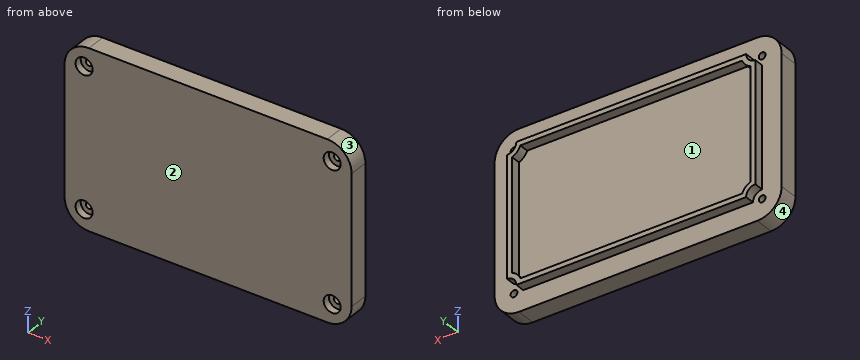
from build123d import *

# Parameters (mm, degrees)
SKETCH1_R           = 1.4
BOSS_EXTRUDE1_DEPTH = 8
BOSS_EXTRUDE2_DEPTH = 8
BOSS_EXTRUDE3_DEPTH = 4
SKETCH4_R           = 3.5
CUT_EXTRUDE1_DEPTH  = 3


with BuildPart() as part:
    # Sketch1 → Boss-Extrude1 (new body)
    with BuildSketch(Plane(origin=(0, 0, 0), x_dir=(1, 0, 0), z_dir=(0, 1, 0))):
        with BuildLine():
            ThreePointArc((-49, 36.5), (-56.071067812, 33.571067812), (-59, 26.5))
            Line((-59, 26.5), (-59, -26.5))
            ThreePointArc((-59, -26.5), (-56.071067812, -33.571067812), (-49, -36.5))
            Line((-49, -36.5), (49, -36.5))
            ThreePointArc((49, -36.5), (56.071067812, -33.571067812), (59, -26.5))
            Line((59, -26.5), (59, 26.5))
            ThreePointArc((59, 26.5), (56.071067812, 33.571067812), (49, 36.5))
            Line((49, 36.5), (-49, 36.5))
        make_face()
        with Locations(Location((-51, -28.5, 0), (0, 0, 270))):
            Circle(SKETCH1_R, mode=Mode.SUBTRACT)
        with Locations(Location((51, -28.5, 0), (0, 0, 270))):
            Circle(SKETCH1_R, mode=Mode.SUBTRACT)
        with Locations(Location((-51, 28.5, 0), (0, 0, 270))):
            Circle(SKETCH1_R, mode=Mode.SUBTRACT)
        with BuildLine():
            Line((43.828427125, -28.5), (-43.828427125, -28.5))
            Line((-43.828427125, -28.5), (-47.234932778, -28.5))
            ThreePointArc((-47.234932778, -28.5), (-48.337695436, -25.837695436), (-51, -24.734932778))
            Line((-51, -24.734932778), (-51, -21.328427125))
            Line((-51, -21.328427125), (-51, 21.328427125))
            Line((-51, 21.328427125), (-51, 24.734932778))
            ThreePointArc((-51, 24.734932778), (-48.337695436, 25.837695436), (-47.234932778, 28.5))
            Line((-47.234932778, 28.5), (-43.828427125, 28.5))
            Line((-43.828427125, 28.5), (43.828427125, 28.5))
            Line((43.828427125, 28.5), (47.234932778, 28.5))
            ThreePointArc((47.234932778, 28.5), (48.337695436, 25.837695436), (51, 24.734932778))
            Line((51, 24.734932778), (51, 21.328427125))
            Line((51, 21.328427125), (51, -21.328427125))
            Line((51, -21.328427125), (51, -24.734932778))
            ThreePointArc((51, -24.734932778), (48.337695436, -25.837695436), (47.234932778, -28.5))
            Line((47.234932778, -28.5), (43.828427125, -28.5))
        make_face(mode=Mode.SUBTRACT)
        with Locations(Location((51, 28.5, 0), (0, 0, 270))):
            Circle(SKETCH1_R, mode=Mode.SUBTRACT)
    extrude(amount=BOSS_EXTRUDE1_DEPTH)



with BuildPart() as body_2:
    # Sketch2 → Boss-Extrude2 (new body)
    with BuildSketch(Plane(origin=(0, 8, 0), x_dir=(1, 0, 0), z_dir=(0, 1, 0))):
        with BuildLine():
            Line((51, -24.734932778), (51, 24.734932778))
            ThreePointArc((51, 24.734932778), (48.337695436, 25.837695436), (47.234932778, 28.5))
            Line((47.234932778, 28.5), (-47.234932778, 28.5))
            ThreePointArc((-47.234932778, 28.5), (-48.337695436, 25.837695436), (-51, 24.734932778))
            Line((-51, 24.734932778), (-51, -24.734932778))
            ThreePointArc((-51, -24.734932778), (-48.337695436, -25.837695436), (-47.234932778, -28.5))
            Line((-47.234932778, -28.5), (47.234932778, -28.5))
            ThreePointArc((47.234932778, -28.5), (48.337695436, -25.837695436), (51, -24.734932778))
        make_face()
    extrude(amount=-BOSS_EXTRUDE2_DEPTH)


with BuildPart() as part_1:
    add(part.part)

    add(body_2.part)  # Boss-Extrude3 merges body 2
    # Sketch3 → Boss-Extrude3 (add)
    with BuildSketch(Plane(origin=(0, 8, 0), x_dir=(1, 0, 0), z_dir=(0, 1, 0))):
        with BuildLine():
            ThreePointArc((47.234932778, -28.5), (48.337695436, -25.837695436), (51, -24.734932778))
            Line((51, -24.734932778), (51, 24.734932778))
            ThreePointArc((51, 24.734932778), (48.337695436, 25.837695436), (47.234932778, 28.5))
            Line((47.234932778, 28.5), (-45.234932778, 28.5))
            Line((-45.234932778, 28.5), (-47.234932778, 28.5))
            ThreePointArc((-47.234932778, 28.5), (-48.337695436, 25.837695436), (-51, 24.734932778))
            Line((-51, 24.734932778), (-51, -24.734932778))
            ThreePointArc((-51, -24.734932778), (-48.337695436, -25.837695436), (-47.234932778, -28.5))
            Line((-47.234932778, -28.5), (47.234932778, -28.5))
        make_face()
        with BuildLine():
            ThreePointArc((-49, 23.092967535), (-46.923481873, 24.423481873), (-45.592967535, 26.5))
            Line((-45.592967535, 26.5), (45.592967535, 26.5))
            ThreePointArc((45.592967535, 26.5), (46.923481873, 24.423481873), (49, 23.092967535))
            Line((49, 23.092967535), (49, -23.092967535))
            ThreePointArc((49, -23.092967535), (46.923481873, -24.423481873), (45.592967535, -26.5))
            Line((45.592967535, -26.5), (-45.592967535, -26.5))
            ThreePointArc((-45.592967535, -26.5), (-46.923481873, -24.423481873), (-49, -23.092967535))
            Line((-49, -23.092967535), (-49, 23.092967535))
        make_face(mode=Mode.SUBTRACT)
    extrude(amount=BOSS_EXTRUDE3_DEPTH)

    # Sketch4 → Cut-Extrude1 (cut)
    with BuildSketch(Plane.XZ):
        with Locations(Location((-51, 28.5, 0), (0, 0, 270))):
            Circle(SKETCH4_R)
        with Locations(Location((51, 28.5, 0), (0, 0, 90))):
            Circle(SKETCH4_R)
        with Locations(Location((51, -28.5, 0), (0, 0, 270))):
            Circle(SKETCH4_R)
        with Locations(Location((-51, -28.5, 0), (0, 0, 90))):
            Circle(SKETCH4_R)
    extrude(amount=-CUT_EXTRUDE1_DEPTH, mode=Mode.SUBTRACT)


solid = part_1.part
CAD build for the part. Positions are in the model's coordinates, mm. Face numbers are marked on the shaded views. Give positions to 0.01 mm unless a question says otherwise; leave off trailing zeros. Write each loop counter-clockwise with the first axis right and the second up, starting at its lowest first coordinate (ties: lowest second). Pieces come first, ordered by that corner, then holes. Notation, with made-up numbers: M -38.75,87 L -33.75,87 A21 cw -33.75,122 Z; hole C 56,48 d11. An arc over 180 degrees is marked long. Put each result on its own line as item: value. Start each with the question number.
(1) Flat gauge pins, fed straight in: pin 1 Ø3 at (y, z) = (10.5, 10.5) entering from -X; pin 2 Ø2 at (x, y) = (20, 11) entering from +Z; pin 3 Ø2 at (x, z) = (-50.5, 27) entering from -Y. Where does each tip first touch, or does it go through?
(2) Band-saw the part on A-A, the plane y = 10.75. Write the cut outline in (x, z).
(3) Mould opens along Z. For the marked faces 1, 2, 3 and 4 say: +Z half, -Z half, draft (parallel to the pull), parting line (faces both ways), or undercut.
(4) Band-saw the part on C-C, the plane z = -10.5. Write the cut outline in (x, y), and give its area (3 significant figures).
(5) Probe L1, parallel to Z at x = -51, y = 4.35; L2, parallel to Z at x = 20.5, y = 9.75; L3, parallel to X at y = 4.95, z = -28.5. List the from-to ranges inside material, lowest first.
(6) Band-saw the part on B-B, the plane x = -10. Write the cut outline in (y, z).
Response values:
1. pin 1: stops at x = -51
1. pin 2: stops at z = 28.5
1. pin 3: stops at y = 3
2. outline: M -51,-24.73 A3.77 cw -47.23,-28.5 L 47.23,-28.5 A3.77 cw 51,-24.73 L 51,24.73 A3.77 cw 47.23,28.5 L -47.23,28.5 A3.77 cw -51,24.73 Z; hole M -49,-23.09 A5.77 cw -45.59,-26.5 L 45.59,-26.5 A5.77 cw 49,-23.09 L 49,23.09 A5.77 cw 45.59,26.5 L -45.59,26.5 A5.77 cw -49,23.09 Z
3. face 1: undercut
3. face 2: draft
3. face 3: +Z half
3. face 4: -Z half
4. outline: M -59,0 L 59,0 L 59,8 L 51,8 L 51,12 L 49,12 L 49,8 L -49,8 L -49,12 L -51,12 L -51,8 L -59,8 Z
4. area: 960 mm2
5. L1: z = -36.3 to -29.9, -27.1 to 27.1, 29.9 to 36.3
5. L2: z = -28.5 to -26.5, 26.5 to 28.5
5. L3: x = -58.8 to -52.4, -49.6 to 49.6, 52.4 to 58.8
6. outline: M 0,-36.5 L 8,-36.5 L 8,-28.5 L 12,-28.5 L 12,-26.5 L 8,-26.5 L 8,26.5 L 12,26.5 L 12,28.5 L 8,28.5 L 8,36.5 L 0,36.5 Z
